Work out the finished part from the listing and answer in its coordinate system (mm). A direction names the side the tool comes from. Coordinates: 2 decimals unless noted, no trailing zeros. Use a Markdown table: item, result.
from build123d import *

# Parameters (mm, degrees)
BOSS_EXTRUDE1_DEPTH     = 10
CIRPATTERN1_COUNT       = 10
SKETCH1_R               = 11.7825
BOSS_EXTRUDE2_DEPTH     = 10
SKETCH4_R               = 9
SKETCH4_R_2             = 7.5
CUT_EXTRUDE1_DEPTH      = 2
SKETCH4_3_R             = 4
CUT_EXTRUDE2_DEPTH      = 11.0000001
SKETCH5_R               = 9
SKETCH5_R_2             = 7.5
CUT_EXTRUDE3_DEPTH      = 2
FILLET1_R               = 0.5
CHAMFER1_SIZE           = 0.5
CHAMFER2_SIZE           = 0.5
SKETCH6_W               = 3
SKETCH6_H               = 3
CUT_EXTRUDE4_DEPTH      = 11.0000001
CUT_EXTRUDE4_DEPTH_BACK = 1.0000001


with BuildPart() as part:
    # Sketch3 → Boss-Extrude1 (new body)
    with BuildSketch(Plane.XY):
        with BuildLine():
            Line((4.803075617, 13.959368513), (3.833494733, 11.141437267))
            ThreePointArc((3.833494733, 11.141437267), (1.943363276, 11.621129266), (0, 11.7825))
            Line((0, 11.7825), (0, 14.762571073))
            add(Edge.make_bspline(
                [(0, 14.762571073), (0.333518774, 16.315241106), (1.140884964, 17.626707575), (2.241097954, 18.718316804)],
                knots=[0, 0, 0, 0, 0.256830749, 0.256830749, 0.256830749, 0.256830749], degree=3))
            ThreePointArc((2.241097954, 18.718316804), (3.109381242, 18.593806826), (3.970932877, 18.429042191))
            add(Edge.make_bspline(
                [(4.803075617, 13.959368513), (4.992871831, 15.536072798), (4.656124965, 17.038865536), (3.970932877, 18.429042191)],
                knots=[0, 0, 0, 0, 0.256830749, 0.256830749, 0.256830749, 0.256830749], degree=3))
        make_face()
    extrude(amount=BOSS_EXTRUDE1_DEPTH)


with BuildPart() as cirpattern1_1:
    # CirPattern1: pattern copy
    add(part.part.rotate(Axis((0, 0, 0), (0, 0, 1)), 1 * 360 / CIRPATTERN1_COUNT))


with BuildPart() as cirpattern1_2:
    # CirPattern1: pattern copy
    add(part.part.rotate(Axis((0, 0, 0), (0, 0, 1)), 2 * 360 / CIRPATTERN1_COUNT))


with BuildPart() as cirpattern1_3:
    # CirPattern1: pattern copy
    add(part.part.rotate(Axis((0, 0, 0), (0, 0, 1)), 3 * 360 / CIRPATTERN1_COUNT))


with BuildPart() as cirpattern1_4:
    # CirPattern1: pattern copy
    add(part.part.rotate(Axis((0, 0, 0), (0, 0, 1)), 4 * 360 / CIRPATTERN1_COUNT))


with BuildPart() as cirpattern1_5:
    # CirPattern1: pattern copy
    add(part.part.rotate(Axis((0, 0, 0), (0, 0, 1)), 5 * 360 / CIRPATTERN1_COUNT))


with BuildPart() as cirpattern1_6:
    # CirPattern1: pattern copy
    add(part.part.rotate(Axis((0, 0, 0), (0, 0, 1)), 6 * 360 / CIRPATTERN1_COUNT))


with BuildPart() as cirpattern1_7:
    # CirPattern1: pattern copy
    add(part.part.rotate(Axis((0, 0, 0), (0, 0, 1)), 7 * 360 / CIRPATTERN1_COUNT))


with BuildPart() as cirpattern1_8:
    # CirPattern1: pattern copy
    add(part.part.rotate(Axis((0, 0, 0), (0, 0, 1)), 8 * 360 / CIRPATTERN1_COUNT))


with BuildPart() as cirpattern1_9:
    # CirPattern1: pattern copy
    add(part.part.rotate(Axis((0, 0, 0), (0, 0, 1)), 9 * 360 / CIRPATTERN1_COUNT))


with BuildPart() as part_1:
    add(part.part)

    add(cirpattern1_1.part)  # Boss-Extrude2 merges CirPattern1_1

    add(cirpattern1_2.part)  # Boss-Extrude2 merges CirPattern1_2

    add(cirpattern1_3.part)  # Boss-Extrude2 merges CirPattern1_3

    add(cirpattern1_4.part)  # Boss-Extrude2 merges CirPattern1_4

    add(cirpattern1_5.part)  # Boss-Extrude2 merges CirPattern1_5

    add(cirpattern1_6.part)  # Boss-Extrude2 merges CirPattern1_6

    add(cirpattern1_7.part)  # Boss-Extrude2 merges CirPattern1_7

    add(cirpattern1_8.part)  # Boss-Extrude2 merges CirPattern1_8

    add(cirpattern1_9.part)  # Boss-Extrude2 merges CirPattern1_9
    # Sketch1 → Boss-Extrude2 (add)
    with BuildSketch(Plane.XY):
        Circle(SKETCH1_R)
    extrude(amount=BOSS_EXTRUDE2_DEPTH)

    # Sketch4 → Cut-Extrude1 (cut)
    with BuildSketch(Plane.XY.offset(10)):
        Circle(SKETCH4_R)
        Circle(SKETCH4_R_2, mode=Mode.SUBTRACT)
    extrude(amount=-CUT_EXTRUDE1_DEPTH, mode=Mode.SUBTRACT)

    # Sketch4_3 → Cut-Extrude2 (cut, through all)
    with BuildSketch(Plane.XY.offset(10)):
        Circle(SKETCH4_3_R)
    extrude(amount=-CUT_EXTRUDE2_DEPTH, mode=Mode.SUBTRACT)

    # Sketch5 → Cut-Extrude3 (cut)
    with BuildSketch(Plane(origin=(0, 0, 0), x_dir=(-1, 0, 0), z_dir=(0, 0, -1))):
        Circle(SKETCH5_R)
        Circle(SKETCH5_R_2, mode=Mode.SUBTRACT)
    extrude(amount=-CUT_EXTRUDE3_DEPTH, mode=Mode.SUBTRACT)

    # Fillet1
    fillet1_edges = [part_1.edges().sort_by_distance(p)[0] for p in [
        (6.925579735, -9.532242736, 5),
        (3.447410128, -11.26688376, 5),
        (3.833494733, 11.141437267, 5),
        (0, 11.7825, 5),
        (11.205823403, -3.640992736, 5),
        (9.411521493, -7.088763604, 5),
        (11.205823403, 3.640992736, 5),
        (11.780751534, -0.202976689, 5),
        (6.925579735, 9.532242736, 5),
        (9.650134902, 6.760340422, 5),
        (-6.925579735, 9.532242736, 5),
        (-3.447410128, 11.26688376, 5),
        (-11.205823403, 3.640992736, 5),
        (-9.411521493, 7.088763604, 5),
        (-11.205823403, -3.640992736, 5),
        (-11.780751534, 0.202976689, 5),
        (-6.925579735, -9.532242736, 5),
        (-9.650134902, -6.760340422, 5),
        (0, -11.7825, 5),
        (-3.833494733, -11.141437267, 5),
    ]]
    fillet(fillet1_edges, radius=FILLET1_R)

    # Chamfer1
    chamfer1_edges = [part_1.edges().sort_by_distance(p)[0] for p in [
        (-7.5, 0, 10),
        (7.5, 0, 0),
    ]]
    chamfer(chamfer1_edges, length=CHAMFER1_SIZE)

    # Chamfer2
    chamfer2_edges = [part_1.edges().sort_by_distance(p)[0] for p in [
        (-9, 0, 10),
        (9, 0, 0),
    ]]
    chamfer(chamfer2_edges, length=CHAMFER2_SIZE)

    # Sketch6 → Cut-Extrude4 (cut, two sides)
    with BuildSketch(Plane.XY) as cut_extrude4_sk:
        with Locations((0, 4)):
            Rectangle(SKETCH6_W, SKETCH6_H)
    extrude(amount=CUT_EXTRUDE4_DEPTH, mode=Mode.SUBTRACT)
    extrude(cut_extrude4_sk.sketch, amount=-CUT_EXTRUDE4_DEPTH_BACK, mode=Mode.SUBTRACT)


solid = part_1.part
(1) Which of the six approach directions +Z, -Z, +X, -X, +Y, -Y give full straight-line access (tool end or side, diameter ignored) to faces 4 (the flat face through (10.81, -8.14, 4.93)), 5 (the flat face through (-12.84, 4.17, 4.93)), 6 (the flat face through (11.09, 7.77, 4.93)), 7 (the cylindrical face through (18.643, 2.801, 4.93)), 8 (the flat face through (-1.5, 5, 5))?
Conclusion:
| item | result |
|---|---|
| face 4 | +Z, -Z, -Y |
| face 5 | +Z, -Z, -X |
| face 6 | +Z, -Z, +X |
| face 7 | +Z, -Z, +X, +Y |
| face 8 | +Z, -Z |
(2) Straight lines are drawn through the part: L1, parallel to X at y = 1.5, z = 1.5; L2, parallel to X at y = -11, z = 7.75; L3, parallel to Y at x = 10.5, z = 5.75. For each, find the intervals that lie inside material, in ascending order.
Conclusion:
| item | result |
|---|---|
| L1 | -11.69 to -8.87, -7.35 to -3.71, 3.71 to 7.35, 8.87 to 18.3 |
| L2 | -13.63 to -7.99, -4.23 to 7.99 |
| L3 | -7.91 to 5.35, 7.36 to 13.14 |
(3) Given P1, Ø2, axis at y = -14, z = 5.5, coming from the +X side; P2, Ø10, axis at x = 1, y = 14.5, coming from the -Z side; P3, Ø2.5, axis at y = 13.5, z = 6.5, coming from the -X side; P4, Ø3, axis at y = -6.5, z = 8.5, coming from the -X side, each flat-ended and moving along its own axis, determine where each tip first touches the part or whether it passes through.
Conclusion:
| item | result |
|---|---|
| P1 | x = 9.31 |
| P2 | z = 0 |
| P3 | x = -9.31 |
| P4 | x = -11.42 |
(4) Determine the mould class of faces 1 (the flat face through (-11.09, -7.77, 4.93)), 2 (the flat face through (2, 7.4, 2)), 3 (the flat face through (-1, 10, 0)) for opening direction X: pulls with the +X half, pulls with the -X half, needs draft (parallel to the pull), parting line crosses it, or undercut.
Conclusion:
| item | result |
|---|---|
| face 1 | pulls with the -X half |
| face 2 | undercut |
| face 3 | needs draft |
